from build123d import *

# Parameters (mm, degrees)
F0_W      = 114.3
F0_H      = 152.4
F1_DEPTH  = 82.55
F2_W      = 60.96
F2_H      = 95.25
F3_DEPTH  = 76.2
F4_R      = 11.734963
F5_DEPTH  = 75.184
F6_W      = 60.96
F6_H      = 38.932147
F7_DEPTH  = 76.2
F8_W      = 88.9
F8_H      = 38.1
F9_DEPTH  = 44.45
F10_W     = 55.88
F10_H     = 33.02
F10_H_2   = 38.1
F11_DEPTH = 43.18
F12_R     = 2.5
F13_DEPTH = 33.02
F14_R     = 2.5
F14_R_2   = 2.3
F15_DEPTH = 2.54
F17_DEPTH = 45.72
F19_DEPTH = 45.72
F20_R     = 3.2
F21_DEPTH = 1.5875
F22_W     = 41.402
F22_H     = 69.85
F23_DEPTH = 40.64


with BuildPart() as f1:
    # F0 (on Top) → F1 (new body)
    with BuildSketch(Plane.XY):
        with Locations((-57.15, 76.2)):
            Rectangle(F0_W, F0_H)
    extrude(amount=-F1_DEPTH)

    # F2 (on face) → F3 (cut)
    with BuildSketch(Plane.XY):
        with Locations((-36.83, 53.975)):
            Rectangle(F2_W, F2_H)
    extrude(amount=-F3_DEPTH, mode=Mode.SUBTRACT)

    # F4 (on face) → F5 (cut)
    with BuildSketch(Plane.YZ):
        with Locations((50.100744, 0)):
            Circle(F4_R)
    extrude(amount=-F5_DEPTH, mode=Mode.SUBTRACT)

    # F6 (on face) → F7 (cut)
    with BuildSketch(Plane.XY):
        with Locations((-36.83, 126.583926)):
            Rectangle(F6_W, F6_H)
    extrude(amount=-F7_DEPTH, mode=Mode.SUBTRACT)

    # F8 (on face) → F9 (cut)
    with BuildSketch(Plane(origin=(-114.3, 0, 0), x_dir=(0, -1, 0), z_dir=(-1, 0, 0))):
        with Locations((-44.45, -63.5)):
            Rectangle(F8_W, F8_H)
    extrude(amount=-F9_DEPTH, mode=Mode.SUBTRACT)

    # F10 (on face) → F11 (cut)
    with BuildSketch(Plane(origin=(-114.3, 0, 0), x_dir=(0, -1, 0), z_dir=(-1, 0, 0))):
        with Locations((-121.190508, -19.685)):
            Rectangle(F10_W, F10_H)
        with Locations((-121.190508, -60.325)):
            Rectangle(F10_W, F10_H_2)
    extrude(amount=-F11_DEPTH, mode=Mode.SUBTRACT)

    # F12 (on face) → F13 (join)
    with BuildSketch(Plane(origin=(0, 0, -44.45), x_dir=(1, 0, 0), z_dir=(0, 0, -1))):
        with Locations((-109.26, -5.04)):
            Circle(F12_R)
    extrude(amount=F13_DEPTH)

    # F14 (on face) → F15 (join)
    with BuildSketch(Plane(origin=(0, 0, -77.47), x_dir=(1, 0, 0), z_dir=(0, 0, -1))):
        with Locations((-109.26, -5.04)):
            Circle(F14_R)
        with Locations((-109.26, -5.04)):
            Circle(F14_R_2, mode=Mode.SUBTRACT)
    extrude(amount=F15_DEPTH)

    # F16 (on face) → F17 (cut)
    with BuildSketch(Plane(origin=(-114.3, 0, 0), x_dir=(0, -1, 0), z_dir=(-1, 0, 0))):
        Polygon((-91.980508, -16.831285), (-91.980508, -18.101285), (-93.250508, -18.101285), (-93.250508, -20.641285), (-91.980508, -20.641285), (-91.980508, -21.911285), (-90.075508, -21.911285), (-90.075508, -16.831285), align=None)
    extrude(amount=-F17_DEPTH, mode=Mode.SUBTRACT)

    # F18 (on face) → F19 (cut)
    with BuildSketch(Plane(origin=(-114.3, 0, 0), x_dir=(0, -1, 0), z_dir=(-1, 0, 0))):
        Polygon((-91.973217, -57.956658), (-91.973217, -59.226658), (-93.250508, -59.226658), (-93.250508, -61.766658), (-91.973217, -61.766658), (-91.973217, -63.036658), (-90.068217, -63.036658), (-90.068217, -57.956658), align=None)
    extrude(amount=-F19_DEPTH, mode=Mode.SUBTRACT)

    # F20 (on face) → F21 (cut)
    with BuildSketch(Plane(origin=(-71.12, 0, 0), x_dir=(0, -1, 0), z_dir=(-1, 0, 0))):
        with Locations((-121.190508, -20.574)):
            Circle(F20_R)
        with Locations((-121.190508, -60.325)):
            Circle(F20_R)
    extrude(amount=-F21_DEPTH, mode=Mode.SUBTRACT)

    # F22 (on face) → F23 (cut)
    with BuildSketch(Plane.XY):
        with Locations((-90.600921, 41.275)):
            Rectangle(F22_W, F22_H)
    extrude(amount=-F23_DEPTH, mode=Mode.SUBTRACT)

    # F24 (on face) → F25 (revolve, cut)
    with BuildSketch(Plane.XZ):
        with BuildLine():
            Line((-7.48795, -4.186609), (-2.48795, -4.186609))
            ThreePointArc((-2.48795, -4.186609), (-4.98795, -1.686609), (-7.48795, -4.186609))
        make_face()
    revolve(axis=Axis((-4.98795, 0, -4.186609), (1, 0, 0)), mode=Mode.SUBTRACT)


solid = f1.part
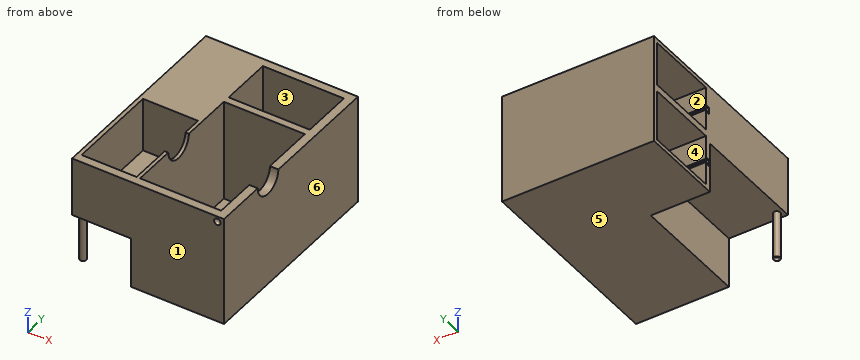
Can you work these out from the model? Positions are in its coordinate system, mm. Face numbers are marked on the shaded views. A direction names the side the tool comes from. Round coordinates to 2 decimals unless told otherwise and drop trailing zeros. Write each loop counter-clockwise with the first axis right and the second up, starting at its lowest first coordinate (ties: lowest second). Pieces come first, ordered by that corner, then holes. Notation, with made-up numbers: M 44,70 L 55,70 A21 ccw 55,109 Z; hole C -22.5,55.5 d8. An arc over 180 degrees is marked long. Use a Markdown table: item, result.
Item 1: I want a section at C-C (x = -35). List the corners of the cut face in (y, z) for me.
Found:
| item | result |
|---|---|
| outline | M 0,-82.55 L 152.4,-82.55 L 152.4,0 L 146.05,0 L 146.05,-76.2 L 107.12,-76.2 L 107.12,0 L 101.6,0 L 101.6,-76.2 L 6.35,-76.2 L 6.35,0 L 0,0 Z |
Item 2: I want a section at A-A (z = -69). List the corners of the cut face in (x, y) for me, and give its area (3 significant figures).
Found:
| item | result |
|---|---|
| outline | M -114.3,88.9 L -69.85,88.9 L -69.85,0 L 0,0 L 0,152.4 L -114.3,152.4 L -114.3,149.13 L -71.12,149.13 L -71.12,93.25 L -114.3,93.25 Z; C -109.26,5.04 d5; hole M -67.31,6.35 L -6.35,6.35 L -6.35,101.6 L -67.31,101.6 Z; hole M -67.31,107.12 L -6.35,107.12 L -6.35,146.05 L -67.31,146.05 Z |
| area | 2,890 mm2 |
Item 3: Which directions (+Z, -Z, +X, -X, +Y, -Y) give clear straight access to the entire face, cutting with the end or side of a thin tool? Please do the marked faces 1, 2 and 3.
Found:
| item | result |
|---|---|
| face 1 | +Z, -Z, +X, -X, -Y |
| face 2 | -X |
| face 3 | +Z |
Item 4: I want a section at B-B (x = -99). State how many separate pieces and enclosed holes the cut face has, and give its area (3 significant figures).
Found:
| item | result |
|---|---|
| separate pieces | 1 |
| enclosed holes | 2 |
| area | 2,350 mm2 |
Item 5: We'd pull the mould along Z, two halves only. Please class the marked faces 4, 5 and 6: released by +Z, released by -Z, zero draft, split by the parting line, or undercut.
Found:
| item | result |
|---|---|
| face 4 | undercut |
| face 5 | released by -Z |
| face 6 | zero draft |
Item 6: For pin 1 Ø6 at (y, z) = (38.5, -52) entering from -X; pin 2 Ø5 at (x, z) = (-88.5, -64.5) entering from -Y; pin 3 Ø3 at (x, y) = (-34, 100) entering from +Z, each with a flat end and sliding along its axis, tell me the tip position at first contact or that it passes through.
Found:
| item | result |
|---|---|
| pin 1 | stops at x = -69.85 |
| pin 2 | stops at y = 88.9 |
| pin 3 | stops at z = -76.2 |
Item 7: If I drill on line 1 along Y through (x, z) = (-44, -31.5); line 2 along X through (y, z) = (5.04, -79.05); line 3 along Y through (x, z) = (-109.26, -79.3), over which ranges is the centre line in solid material (lowest first)? Write a range as [from, to].
Found:
| item | result |
|---|---|
| line 1 | y = [0, 6.35], [101.6, 107.12], [146.05, 152.4] |
| line 2 | x = [-111.76, -111.56], [-106.96, -106.76], [-69.85, 0] |
| line 3 | y = [2.54, 2.74], [7.34, 7.54], [88.9, 93.25], [149.13, 152.4] |
